Input: part model. Units: mm. Frame: model coordinates. A direction names the side the tool comes from. Give positions to 0.01 mm unless a question says otherwise; leave off trailing zeros. Order: outer loops, then holes, each group sorted by start corner. A loop starts at its lowest first (then second) coordinate and runs counter-clockwise, first axis right, second up. Notation, with made-up numbers: M 27,4.5 L 76,4.5 A16 cw 76,29.5 Z; hole C 62,48 d3. An arc over 180 degrees is marked long. Use a Markdown table: item, result.
from build123d import *

# Parameters (mm, degrees)
F1_DEPTH = 8.509
F3_DEPTH = 3.784
F5_DEPTH = 3.784


with BuildPart() as f1:
    # F0 (on Front) → F1 (new body, symmetric)
    with BuildSketch(Plane.XZ):
        with BuildLine():
            ThreePointArc((-22.3393, 0), (0, 22.3393), (22.3393, 0))
            Line((22.3393, 0), (23.8125, 0))
            ThreePointArc((23.8125, 0), (0, 23.8125), (-23.8125, 0))
            Line((-23.8125, 0), (-22.3393, 0))
        make_face()
    extrude(amount=F1_DEPTH, both=True)

    # F2 (on face) → F3 (cut)
    with BuildSketch(Plane.XZ.offset(8.509)):
        with BuildLine():
            Line((-24.2808054107, 0), (-22.3393, 0))
            ThreePointArc((-22.3393, 0), (-22.1925007591, 2.5568016248), (-21.7540323731, 5.08))
            Line((-21.7540323731, 5.08), (-23.6446719547, 5.5215033775))
            ThreePointArc((-23.6446719547, 5.5215033775), (-24.1212477924, 2.7790135535), (-24.2808054107, 0))
        make_face()
    extrude(amount=-F3_DEPTH, mode=Mode.SUBTRACT)

    # F4 (on face) → F5 (join, through all)
    with BuildSketch(Plane.XZ.offset(8.509)):
        Polygon((-21.7540323731, 5.08), (-23.1886357568, 5.4150095097), (-24.6253, 0), (-23.101814744, 0), align=None)
    extrude(amount=-F5_DEPTH)


solid = f1.part
1) Material intervals for line 1 (X direction, y = -4.5, z = 9); line 2 (X direction, y = 4, z = 11.25); line 3 (Z direction, x = 2, y = 6.25), sorted ascending. Write a range as from..to.
Response values:
| item | result |
|---|---|
| line 1 | x = -22.05..-20.45, 20.45..22.05 |
| line 2 | x = -20.99..-19.3, 19.3..20.99 |
| line 3 | z = 22.25..23.73 |
2) Cut plane A-A on y = 5.5. Return loops of the section in (x, z) (1 decimal), and give its area (3 significant figures).
Response values:
| item | result |
|---|---|
| outline | M -23.8,0 L -22.3,0 A22.3 cw 22.3,0 L 23.8,0 A23.8 ccw Z |
| area | 107 mm² |
3) Reachability of faces 1 (the face through (-22.44, -6.64, 2.5)), 2 (the face through (-24, -4.725, 1)), 3 (the face through (23, 0, 0)) from +Z, -Z, +X, -X, +Y, -Y: full face, straight path, thin tool, end or side. Return the list, or none.
Response values:
| item | result |
|---|---|
| face 1 | -Z, -Y |
| face 2 | +Z, -X, +Y |
| face 3 | -Z, +X, -X, +Y, -Y |
4) First-contact query: pin 1 Ø6 at (y, z) = (-4.5, 11.5) entering from -X; pin 2 Ø1.5 at (y, z) = (0.5, 19) entering from -X; pin 3 Ø6 at (y, z) = (0.5, 4.5) entering from -X. Flat tips, straight axial feed; report the tip coordinate or a pass-through.
Response values:
| item | result |
|---|---|
| pin 1 | stops at x = -22.24 |
| pin 2 | stops at x = -15.3 |
| pin 3 | stops at x = -23.77 |
5) Cut plane B-B on x = 0. Return loops of the section in (y, z), and give its area (3 significant figures).
Response values:
| item | result |
|---|---|
| outline | M -8.51,22.34 L 8.51,22.34 L 8.51,23.81 L -8.51,23.81 Z |
| area | 25.1 mm² |
